Design review of the part shown in the three views and the two pictorial views. Dimensions are in mm from the part's minimum x, y and z. Coordinates: 2 decimals unless noted, no trailing zeros. Loops run counter-clockwise (first coordinate to the right, second up) from the corner with the lowest first, then second, coordinate; pieces in that order, holes last. Notation, with made-up numbers: M -19,42 L 20,42 A21 ccw 20,63 Z; hole C 78,11 d11. An arc over 180 degrees is marked long. Use CSV: the item, a comma, the result in double quotes. Start each with the question number.
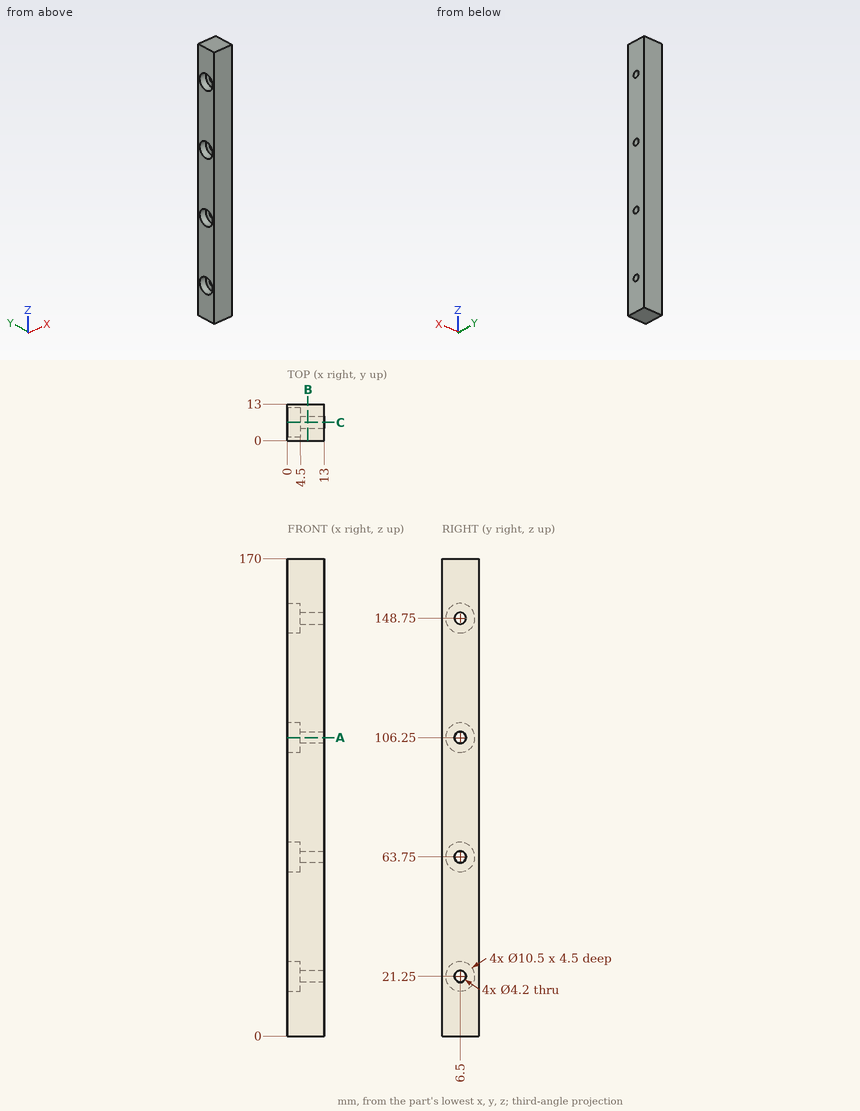
1. To check wall thickness, follow line 1 along Y through (x, z) = (10, 21.25); line 2 along Z through (x, y) = (11, 5.5); line 3 along Z through (x, y) = (1, 10). State the ranges of each line that lie inside material, in increasing order.
2. Add section C-C (y = 6.5). Give the number of separate pieces and of enclosed holes in the cut face, plus the area to 3 significant figures.
3. Insertion check: pin 1 Ø3 at (y, z) = (8, 22) entering from -X; pin 2 Ø5.5 at (y, z) = (6.5, 106.25) entering from +X. Each pin has a flat end and moves straight along its axis. Give the tip position at first contact, or say it passes through.
4. Add section B-B (x = 7.25). Write out the cut boundary in (y, z), plus the area to 3 significant figures.
5. Add section A-A (z = 106.25). Write out the cut boundary in (x, y).
Solved:
1,line 1,"y = 0 to 4.4, 8.6 to 13"
1,line 2,"z = 0 to 19.4, 23.1 to 61.9, 65.6 to 104.4, 108.1 to 146.9, 150.6 to 170"
1,line 3,"z = 0 to 17.34, 25.16 to 59.84, 67.66 to 102.34, 110.16 to 144.84, 152.66 to 170"
2,separate pieces,"5"
2,enclosed holes,"0"
2,area,"1,880 mm^2"
3,pin 1,"stops at x = 4.5"
3,pin 2,"stops at x = 13"
4,outline,"M 0,0 L 13,0 L 13,170 L 0,170 Z; hole C 6.5,21.25 d4.2; hole C 6.5,63.75 d4.2; hole C 6.5,106.25 d4.2; hole C 6.5,148.75 d4.2"
4,area,"2,150 mm^2"
5,outline,"M 0,0 L 13,0 L 13,4.4 L 4.5,4.4 L 4.5,1.25 L 0,1.25 Z; M 0,11.75 L 4.5,11.75 L 4.5,8.6 L 13,8.6 L 13,13 L 0,13 Z"
